from build123d import *

# Parameters (mm, degrees)
F0_W     = 100
F0_H     = 65
F1_DEPTH = 18
F2_W     = 18
F2_H     = 32.5
F3_DEPTH = 30
F4_DEPTH = 30
F6_DEPTH = 25
F7_DEPTH = 43


with BuildPart() as f1:
    # F0 (on Front) → F1 (new body)
    with BuildSketch(Plane.XZ):
        Rectangle(F0_W, F0_H)
    extrude(amount=-F1_DEPTH)

    # F2 (on face) → F3 (join)
    with BuildSketch(Plane.XZ):
        with Locations((-25.2264994979, -16.25)):
            Rectangle(F2_W, F2_H)
    extrude(amount=F3_DEPTH)

    # F2 (on face) → F4 (join)
    with BuildSketch(Plane.XZ):
        with Locations((19.9700337052, -16.25)):
            Rectangle(F2_W, F2_H)
    extrude(amount=F4_DEPTH)

    # F5 (on face) → F6 (join)
    with BuildSketch(Plane.XZ):
        Polygon((-34.2264994979, -32.5), (-34.2264994979, -32.4203260243), (-34.2264994979, 0), (-34.2264994979, 32.5), (-50, 32.5), (-50, -32.5), align=None)
    extrude(amount=F6_DEPTH)

    # F7 (cut): a face of the model
    f7_faces = [f1.faces().sort_by_distance(p)[0] for p in [
        (-42.1132497489, -25, 0),
    ]]
    extrude(f7_faces, amount=-F7_DEPTH, mode=Mode.SUBTRACT)


solid = f1.part
Work out the finished part from the listing and answer in its coordinate system (mm). A direction names the side the tool comes from. Round coordinates to 2 decimals unless told otherwise and drop trailing zeros. Write each loop counter-clockwise with the first axis right and the second up, starting at its lowest first coordinate (ties: lowest second). Pieces come first, ordered by that corner, then holes.
1) A cutting plane is placed at A-A (y = -17.5). Give the vertices of the cut face in (x, z).
2) A cutting plane is placed at D-D (x = 39.5). Give the vertices of the cut face in (y, z), plus the area to 3 significant figures.
3) Given pin 1 Ø9 at (y, z) = (-13, -11.5) entering from +X; pin 2 Ø14.5 at (x, y) = (24.5, -13) entering from +Z; pin 3 Ø5 at (x, z) = (-19, 9.5) entering from -Y, each flat-ended and moving along its own axis, determine where each tip first touches the part or whether it passes through.
4) Straight lines are drawn through the part: line 1 (X direction, y = -8, z = -5); line 2 (Z direction, x = -24, y = -19); line 3 (Y direction, x = 22, z = 6.5). For each, find the intervals that lie inside material, in ascending order.
5) A tool of negligible diameter and unlimited length cuts with its end or side. For faces 4 (the flat face through (20, -15, 0)), 5 (the flat face through (7, 18, 0)), 6 (the flat face through (28.97, -15, -16)), 7 (the flat face through (-16.226, -15, -16)), from which of +Z, -Z, +X, -X, +Y, -Y can it reach the whole face along a straight path? Write none if from no direction.
6) A cutting plane is placed at C-C (x = -27.5). Give the vertices of the cut face in (y, z).
7) The mould has two halves that part along X. Classify faces 1 (the flat face through (50, 9, 0)), 2 (the flat face through (10.97, -15, -16)), 3 (the flat face through (7, 4, -32.5)): pulls with the +X half, pulls with the -X half, needs draft (parallel to the pull), parting line crosses it, or undercut.
8) A cutting plane is placed at B-B (z = -15.5). Give the vertices of the cut face in (x, y), plus the area to 3 significant figures.
Completed:
1. outline: (-34.23, -32.5) - (-16.23, -32.5) - (-16.23, 0) - (-34.23, 0) - close; (10.97, -32.5) - (28.97, -32.5) - (28.97, 0) - (10.97, 0) - close
2. outline: (0, -32.5) - (18, -32.5) - (18, 32.5) - (0, 32.5) - close
2. area: 1,170 mm2
3. pin 1: stops at x = 28.97
3. pin 2: stops at z = 0
3. pin 3: stops at y = 0
4. line 1: x = -34.23 to -16.23, 10.97 to 28.97
4. line 2: z = -32.5 to 0
4. line 3: y = 0 to 18
5. face 4: +Z, +X, -X, -Y
5. face 5: +Z, -Z, +X, -X, +Y
5. face 6: +Z, -Z, +X, -Y
5. face 7: +Z, -Z, -Y
6. outline: (-30, -32.5) - (18, -32.5) - (18, 32.5) - (0, 32.5) - (0, 0) - (-30, 0) - close
7. face 1: pulls with the +X half
7. face 2: undercut
7. face 3: needs draft
8. outline: (-34.23, -30) - (-16.23, -30) - (-16.23, 0) - (10.97, 0) - (10.97, -30) - (28.97, -30) - (28.97, 0) - (50, 0) - (50, 18) - (-34.23, 18) - close
8. area: 2,600 mm2
